Input: part model. Units: mm. Frame: model coordinates. Round coordinates to 2 decimals unless told otherwise and drop trailing zeros. Loops run counter-clockwise (first coordinate to the right, second up) from the corner with the lowest first, then second, coordinate; pieces in that order, holes last. Notation, with made-up numbers: M 75,70.25 L 110,70.25 A28 ccw 110,92.25 Z; hole C 57,87.25 d8. An arc over 180 degrees is marked long. Return JSON: item names as keys, results as strings. Group by question number.
1) Material intervals for line 1 (X direction, y = 2.8, z = 0); line 2 (Z direction, x = -1.5, y = 4.6), sorted ascending. Write a range as from..to.
2) Section A-A (x = 0). Output: boundary loops of the cut face in (y, z), plus the area to 3 significant figures.
3) Section C-C (y = 1.05). Output: boundary loops of the cut face in (x, z).
4) Section B-B (z = 0). Output: boundary loops of the cut face in (x, y), plus the area to 3 significant figures.
5) Mould query, pull axis X, two halves, no side actions, for faces 1 (the face through (-0.867, 1.972, 3.905)), 2 (the face through (-0.2, 5, 5.4)), 3 (the face through (-10.316, 2.472, 7.91)). Classes: +X half, -X half, draft (parallel to the pull), parting line (faces both ways), or undercut.
from build123d import *

# Parameters (mm, degrees)
SKETCH1_R           = 13
SKETCH1_R_2         = 4
BOSS_EXTRUDE1_DEPTH = 5
CHAMFER1_SIZE       = 1
FILLET1_R           = 0.5


with BuildPart() as part:
    # Sketch1 → Boss-Extrude1 (new body)
    with BuildSketch(Plane(origin=(0, 0, 0), x_dir=(1, 0, 0), z_dir=(0, 1, 0))):
        Circle(SKETCH1_R)
        Circle(SKETCH1_R_2, mode=Mode.SUBTRACT)
    extrude(amount=BOSS_EXTRUDE1_DEPTH)

    # Chamfer1
    chamfer1_edges = [part.edges().sort_by_distance(p)[0] for p in [
        (-4, 5, 0),
    ]]
    chamfer(chamfer1_edges, length=CHAMFER1_SIZE)

    # Fillet1
    fillet1_edges = [part.edges().sort_by_distance(p)[0] for p in [
        (-13, 0, 0),
        (-13, 5, 0),
    ]]
    fillet(fillet1_edges, radius=FILLET1_R)


solid = part.part
Returned:
{
 "1": {"line 1": "x = -13..-4, 4..13", "line 2": "z = -12.9..-4.35, 4.35..12.9"},
 "2": {"outline": "M 0,-12.5 A0.5 ccw 0.5,-13 L 4.5,-13 A0.5 ccw 5,-12.5 L 5,-5 L 4,-4 L 0,-4 Z; M 0,4 L 4,4 L 5,5 L 5,12.5 A0.5 ccw 4.5,13 L 0.5,13 A0.5 ccw 0,12.5 Z", "area": "88.8 mm^2"},
 "3": {"outline": "C 0,0 d26; hole C 0,0 d8"},
 "4": {"outline": "M -13,0.5 A0.5 ccw -12.5,0 L -4,0 L -4,4 L -5,5 L -12.5,5 A0.5 ccw -13,4.5 Z; M 4,0 L 12.5,0 A0.5 ccw 13,0.5 L 13,4.5 A0.5 ccw 12.5,5 L 5,5 L 4,4 Z", "area": "88.8 mm^2"},
 "5": {"face 1": "undercut", "face 2": "draft", "face 3": "parting line"}
}
